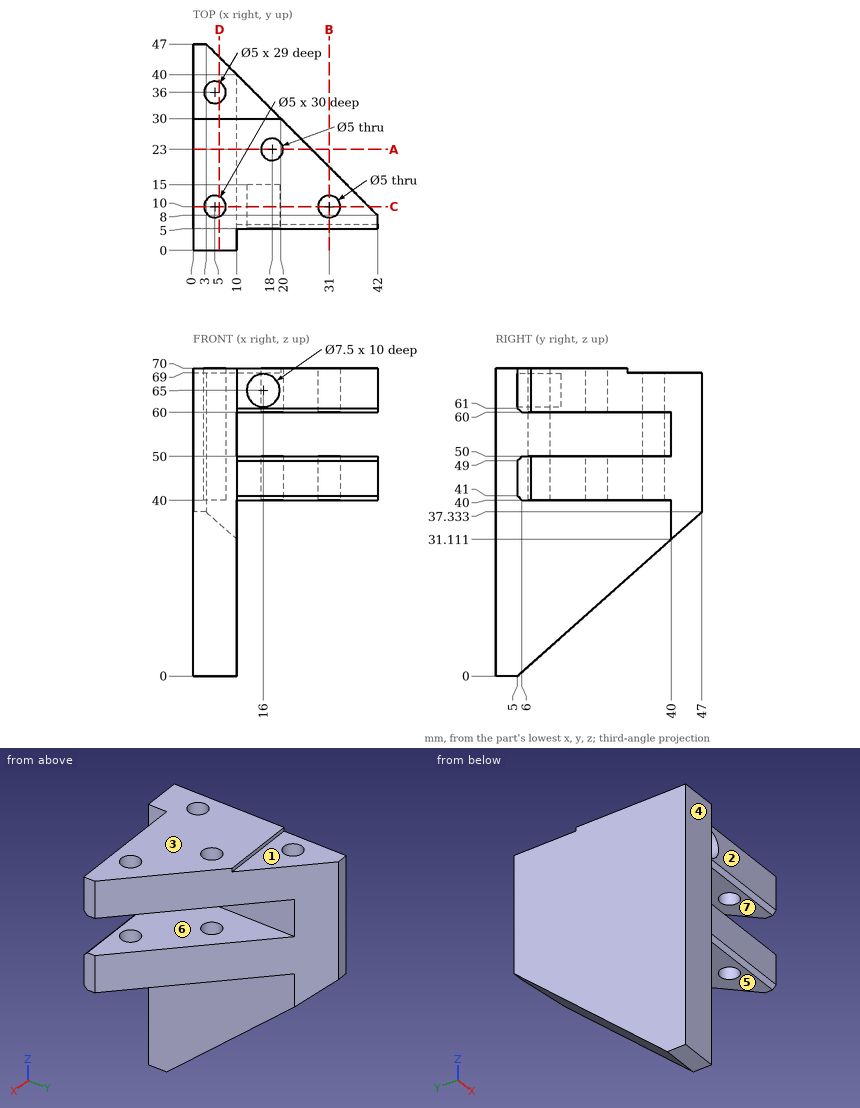
The figure shows three views and two pictorial views of one solid part (mm, origin at its lowest corner). Answer the questions. A direction names the side the tool comes from. Give positions to 0.01 mm unless a question says otherwise; leave off trailing zeros. Loops run counter-clockwise (first coordinate to the right, second up) from the corner with the lowest first, then second, coordinate; pieces in that order, holes last. Notation, with made-up numbers: (33, -24) - (62, -24) arc R31 ccw to (62, 14) - close; hole circle Ø5 at (-35, -31.75). An arc over 180 degrees is marked (long way). Answer in a Markdown table with one row per item.
(1) Consider L1, parallel to Z at x = 15, y = 24; L2, parallel to Y at x = 5, z = 60.75; L3, parallel to Z at x = 18.5, y = 5.5 (1 decimal). Determine where each line is inside the solid, lowest interval first. Write a range as [from, to].
Results list:
| item | result |
|---|---|
| L1 | z = [40, 50], [60, 70] |
| L2 | y = [0, 7.5], [12.5, 33.5], [38.5, 45] |
| L3 | z = [40.5, 49.5], [60.5, 62.2], [67.8, 70] |
(2) Section A-A (y = 23) is taken. Give the vertices of the cut face in (x, z), and give its area (3 significant figures).
Results list:
| item | result |
|---|---|
| outline | (0, 16) - (10, 16) - (10, 40) - (15.5, 40) - (15.5, 50) - (10, 50) - (10, 60) - (15.5, 60) - (15.5, 70) - (0, 70) - close; (20.5, 40) - (27, 40) - (27, 50) - (20.5, 50) - close; (20.5, 60) - (27, 60) - (27, 70) - (20.5, 70) - close |
| area | 780 mm² |
(3) Section B-B (x = 31) is taken. Give the vertices of the cut face in (y, z).
Results list:
| item | result |
|---|---|
| outline | (5, 41) - (6, 40) - (7.5, 40) - (7.5, 50) - (6, 50) - (5, 49) - close; (5, 61) - (6, 60) - (7.5, 60) - (7.5, 70) - (5, 70) - close; (12.5, 40) - (19, 40) - (19, 50) - (12.5, 50) - close; (12.5, 60) - (19, 60) - (19, 70) - (12.5, 70) - close |
(4) Section D-D (x = 6) is taken. Give the vertices of the cut face in (y, z), and give its area (3 significant figures).
Results list:
| item | result |
|---|---|
| outline | (0, 0) - (5, 0) - (44, 34.67) - (44, 69) - (38.29, 69) - (38.29, 40) - (33.71, 40) - (33.71, 69) - (30, 69) - (30, 70) - (12.29, 70) - (12.29, 40) - (7.71, 40) - (7.71, 70) - (0, 70) - close |
| area | 2,120 mm² |
(5) Section C-C (y = 10) is taken. State how many separate pieces and enclosed holes the cut face has.
Results list:
| item | result |
|---|---|
| separate pieces | 3 |
| enclosed holes | 1 |
(6) A tool of negligible diameter and unlimited length cuts with its end or side. For the marked faces 1, 2 and 3, from which of +Z, -Z, +X, -X, +Y, -Y can it reach the whole face along a straight path? Write none if from no direction.
Results list:
| item | result |
|---|---|
| face 1 | +Z, +X, -X, +Y |
| face 2 | +Z, -Z, +X, -Y |
| face 3 | +Z, +X, -X, +Y, -Y |
(7) For a pull along Z with two mould halves and no side action, classify the marked faces 4, 5, 6 and 7 as pulls with the +Z half, pulls with the -Z half, needs draft (parallel to the pull), parting line crosses it, or undercut.
Results list:
| item | result |
|---|---|
| face 4 | needs draft |
| face 5 | pulls with the -Z half |
| face 6 | undercut |
| face 7 | undercut |
(8) Flat-ended cylindrical pins translate along their axes: pin 1 Ø8 at (x, y) = (31, 10) entering from -Z; pin 2 Ø12 at (x, z) = (22, 38.5) entering from -Y; pin 3 Ø18.5 at (x, y) = (13, 39.5) entering from +Z. Find the tip coordinate at first contact, or state that the pin passes through.
Results list:
| item | result |
|---|---|
| pin 1 | stops at z = 40 |
| pin 2 | stops at y = 5 |
| pin 3 | stops at z = 69 |
